Geometry check sheet. Reference: the model listing, model coordinates, mm. A direction names the side the tool comes from. Round coordinates to 2 decimals unless told otherwise and drop trailing zeros. Order: outer loops, then holes, each group sorted by start corner. A loop starts at its lowest first (then second) coordinate and runs counter-clockwise, first axis right, second up. Notation, with made-up numbers: (77.25, 23.5) - (110.25, 23.5) arc R21 cw to (110.25, 28.5) - close; hole circle Ø8 at (29.25, -12.75). An arc over 180 degrees is marked (long way). Use a Markdown table: item, result. Add a question column.
(1) Mould release check, pull along Y, two halves, no side actions. Record for faces 4 (the face through (7, 44, -15)), 5 (the face through (-2, 3, 0)), 6 (the face through (14, 143, 0)): released by +Y, released by -Y, zero draft, split by the parting line, or undercut.
(2) Section check D-D on y = 10. Record the boundary of the cut face in (x, z), then the cut area to 3 significant figures.
(3) Section check B-B on z = 0. Record the boundary of the cut face in (x, y).
(4) Section check A-A on y = 140.5. Record the boundary of the cut face in (x, z).
(5) Access from +Z, -Z, +X, -X, +Y, -Y to the whole of each face (thin tool, end or side, straight path). Record for faces 1 (the face through (-1.31, 29.87, 13.52)), 2 (the face through (5, 18, -12)), 3 (the face through (14, 87, -7.75)).
(6) Gauge pin test, flat ends, axial feed: P1, Ø6, axis at y = 129.5, z = -4, coming from the +X side (3 decimals); P2, Ø3, axis at y = 91, z = -8.5, coming from the -X side; P3, Ø2, axis at x = -8.5, z = -6.5, coming from the +Y side. Record the tip position at first contact, or that the pin passes through.
(7) Section check C-C on x = -9. Record the boundary of the cut face in (y, z).
(8) Thickness scan on line 1 along Z through (x, y) = (-2, 17.5); line 2 along X through (y, z) = (1.2, -9); line 3 along X through (y, z) = (16, -4.5). Record the ranges inside material, lowest first. Write a range as [from, to].
```python
from build123d import *

# Parameters (mm, degrees)
ESBO_O1_W                = 30
ESBO_O1_H                = 30
ESBO_O1_R                = 1.55
RESSALTO_EXTRUS_O1_DEPTH = 3
ESBO_O2_W                = 3
ESBO_O2_H                = 30
RESSALTO_EXTRUS_O2_DEPTH = 153
ESBO_O3_R                = 1.55
ESBO_O3_W                = 15.5
ESBO_O3_H                = 111
CORTE_EXTRUS_O1_DEPTH    = 153
RESSALTO_EXTRUS_O3_DEPTH = 3
RESSALTO_EXTRUS_O4_DEPTH = 3


with BuildPart() as part:
    # Esboço1 → Ressalto-extrusão1 (new body)
    with BuildSketch(Plane(origin=(0, 0, 0), x_dir=(1, 0, 0), z_dir=(0, 1, 0))):
        Rectangle(ESBO_O1_W, ESBO_O1_H)
        with Locations(Location((-9, -7, 0), (0, 0, 270))):
            Circle(ESBO_O1_R, mode=Mode.SUBTRACT)
        with Locations(Location((7, 9, 0), (0, 0, 270))):
            Circle(ESBO_O1_R, mode=Mode.SUBTRACT)
    extrude(amount=RESSALTO_EXTRUS_O1_DEPTH)

    # Esboço2 → Ressalto-extrusão2 (add)
    with BuildSketch(Plane(origin=(0, 3, 0), x_dir=(1, 0, 0), z_dir=(0, 1, 0))):
        with Locations((13.5, 0)):
            Rectangle(ESBO_O2_W, ESBO_O2_H)
    extrude(amount=RESSALTO_EXTRUS_O2_DEPTH)

    # Esboço3 → Corte-extrusão1 (cut)
    with BuildSketch(Plane(origin=(15, 0, 0), x_dir=(0, 0, -1), z_dir=(1, 0, 0))):
        with Locations((0, 147)):
            Circle(ESBO_O3_R)
        with Locations((0, 27)):
            Circle(ESBO_O3_R)
        with Locations((0, 87.5)):
            Rectangle(ESBO_O3_W, ESBO_O3_H)
    extrude(amount=-CORTE_EXTRUS_O1_DEPTH, mode=Mode.SUBTRACT)

    # Esboço4 → Ressalto-extrusão3 (add)
    with BuildSketch(Plane.XY.offset(15)):
        Polygon((12, 56), (-15, 3), (12, 3), align=None)
    extrude(amount=-RESSALTO_EXTRUS_O3_DEPTH)

    # Esboço5 → Ressalto-extrusão4 (add)
    with BuildSketch(Plane(origin=(0, 0, -15), x_dir=(-1, 0, 0), z_dir=(0, 0, -1))):
        Polygon((15, 3), (-12, 56), (-12, 3), align=None)
    extrude(amount=-RESSALTO_EXTRUS_O4_DEPTH)


solid = part.part
```
Check sheet entries:
| question | item | result |
|---|---|---|
| 1 | face 4 | zero draft |
| 1 | face 5 | released by +Y |
| 1 | face 6 | undercut |
| 2 | outline | (-11.43, -15) - (15, -15) - (15, 15) - (-11.43, 15) - (-11.43, 12) - (12, 12) - (12, -12) - (-11.43, -12) - close |
| 2 | area | 231 mm2 |
| 3 | outline | (-15, 0) - (15, 0) - (15, 25.45) - (12, 25.45) - (12, 3) - (-15, 3) - close; (12, 28.55) - (15, 28.55) - (15, 32) - (12, 32) - close; (12, 143) - (15, 143) - (15, 145.45) - (12, 145.45) - close; (12, 148.55) - (15, 148.55) - (15, 156) - (12, 156) - close |
| 4 | outline | (12, -15) - (15, -15) - (15, -7.75) - (12, -7.75) - close; (12, 7.75) - (15, 7.75) - (15, 15) - (12, 15) - close |
| 5 | face 1 | +Z, -Z, -X, +Y |
| 5 | face 2 | -X, +Y |
| 5 | face 3 | +X, -X |
| 6 | P1 | passes through |
| 6 | P2 | stops at x = 12 |
| 6 | P3 | stops at y = 3 |
| 7 | outline | (0, -15) - (14.78, -15) - (14.78, -12) - (3, -12) - (3, 5.45) - (0, 5.45) - close; (0, 8.55) - (3, 8.55) - (3, 12) - (14.78, 12) - (14.78, 15) - (0, 15) - close |
| 8 | line 1 | z = [-15, -12], [12, 15] |
| 8 | line 2 | x = [-15, 5.45], [8.55, 15] |
| 8 | line 3 | x = [12, 15] |
